Can you work these out from the model? Positions are in its coordinate system, mm. Face numbers are marked on the shaded views. A direction names the side the tool comes from. Coordinates: 2 decimals unless noted, no trailing zeros. Write each loop counter-clockwise with the first axis right and the second up, starting at its lowest first coordinate (ties: lowest second). Pieces come first, ordered by that corner, then holes. Notation, with made-up numbers: (70.5, -25.5) - (85.5, -25.5) arc R24 ccw to (85.5, 10.5) - close; hole circle Ø7 at (35, 7). An arc over 180 degrees is marked (long way). One line per question, with ' | ' between items. Start each with the question number.
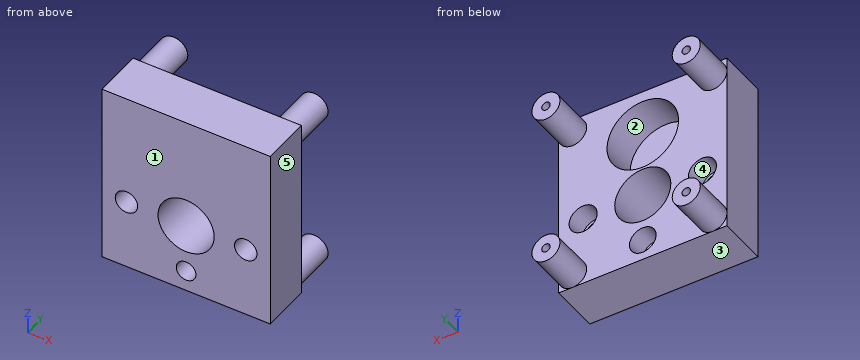
from build123d import *

# Parameters (mm, degrees)
SKETCH_1_W          = 12
SKETCH_1_H          = 13
SKETCH_1_R          = 2
SKETCH_1_R_2        = 0.8
SKETCH_1_R_3        = 0.7
EXTRUDE_1_DEPTH     = 3.5
CUT_EXTRUDE_START   = 3.5
SKETCH_1_3_R        = 1
SKETCH_1_3_R_2      = 0.95
CUT_EXTRUDE_2_DEPTH = 1.5
SKETCH_2_R          = 2.55
CUT_EXTRUDE_5_DEPTH = 2.6
SKETCH_3_R          = 1
EXTRUDE_2_DEPTH     = 3
CUT_EXTRUDE_START_2 = 3
SKETCH_3_3_R        = 0.3
CUT_EXTRUDE_6_DEPTH = 2


with BuildPart() as part:
    # 草图1 → 凸台-拉伸1 (new body)
    with BuildSketch(Plane(origin=(0, 0, 0), x_dir=(1, 0, 0), z_dir=(0, 1, 0))):
        with Locations((0, -1.5)):
            Rectangle(SKETCH_1_W, SKETCH_1_H)
        with Locations(Location((0, 0, 0), (0, 0, 270))):
            Circle(SKETCH_1_R, mode=Mode.SUBTRACT)
        with Locations(Location((-4.25, 0, 0), (0, 0, 270))):
            Circle(SKETCH_1_R_2, mode=Mode.SUBTRACT)
        with Locations(Location((4.25, 0, 0), (0, 0, 270))):
            Circle(SKETCH_1_R_2, mode=Mode.SUBTRACT)
        with Locations(Location((0, 3.5, 0), (0, 0, 270))):
            Circle(SKETCH_1_R_3, mode=Mode.SUBTRACT)
    extrude(amount=EXTRUDE_1_DEPTH)

    # 草图1<3> → 切除-拉伸2 (cut)
    with BuildSketch(Plane(origin=(0, 0, 0), x_dir=(1, 0, 0), z_dir=(0, 1, 0)).offset(CUT_EXTRUDE_START)):
        with Locations(Location((-4.25, 0, 0), (0, 0, 270))):
            Circle(SKETCH_1_3_R)
        with Locations(Location((4.25, 0, 0), (0, 0, 270))):
            Circle(SKETCH_1_3_R)
        with Locations(Location((0, 3.5, 0), (0, 0, 270))):
            Circle(SKETCH_1_3_R_2)
    extrude(amount=-CUT_EXTRUDE_2_DEPTH, mode=Mode.SUBTRACT)

    # 草图2 → 切除-拉伸5 (cut)
    with BuildSketch(Plane(origin=(0, 3.5, 0), x_dir=(1, 0, 0), z_dir=(0, 1, 0))):
        with Locations(Location((0, -4.7, 0), (0, 0, 270))):
            Circle(SKETCH_2_R)
    extrude(amount=-CUT_EXTRUDE_5_DEPTH, mode=Mode.SUBTRACT)

    # 草图3 → 凸台-拉伸2 (add)
    with BuildSketch(Plane(origin=(0, 3.5, 0), x_dir=(1, 0, 0), z_dir=(0, 1, 0))):
        with Locations(Location((-5, -7, 0), (0, 0, 270))):
            Circle(SKETCH_3_R)
        with Locations(Location((5, 4, 0), (0, 0, 90))):
            Circle(SKETCH_3_R)
        with Locations(Location((-5, 4, 0), (0, 0, 90))):
            Circle(SKETCH_3_R)
        with Locations(Location((5, -7, 0), (0, 0, 270))):
            Circle(SKETCH_3_R)
    extrude(amount=EXTRUDE_2_DEPTH)

    # 草图3<3> → 切除-拉伸6 (cut)
    with BuildSketch(Plane(origin=(0, 3.5, 0), x_dir=(1, 0, 0), z_dir=(0, 1, 0)).offset(CUT_EXTRUDE_START_2)):
        with Locations(Location((5, 4, 0), (0, 0, 270))):
            Circle(SKETCH_3_3_R)
        with Locations(Location((-5, -7, 0), (0, 0, 270))):
            Circle(SKETCH_3_3_R)
        with Locations(Location((-5, 4, 0), (0, 0, 270))):
            Circle(SKETCH_3_3_R)
        with Locations(Location((5, -7, 0), (0, 0, 270))):
            Circle(SKETCH_3_3_R)
    extrude(amount=-CUT_EXTRUDE_6_DEPTH, mode=Mode.SUBTRACT)


solid = part.part
(1) Which directions (+Z, -Z, +X, -X, +Y, -Y) give clear straight access to the entire face, cutting with the end or side of a thin tool? Please do the marked faces 1 and 2.
(2) If we section it at D-D on y = 3.25: List the corners of the cut face in (x, z) for me.
(3) If we section it at A-A on x = 0: List the corners of the cut face in (y, z) for me.
(4) If we mould it in two halves opening along X, with no side actions, what happens to the marked faces 3, 4 and 5? For each: +X half, -X half, draft (parallel to the pull), parting line (faces both ways), or undercut.
(5) If I drill on probe 1 along X at (y, z) = (0.8, 0); probe 2 along X at (y, z) = (5.9, -4); probe 3 along Z at (x, y) = (-4.25, 1.5), over which ranges is the centre line in solid material (lowest first)?
(6) If we section it at B-B on y = 5.75: List the corners of the cut face in (x, z) for me, plus the area to 3 significant figures.
(7) I'm going to push flat-ended pins straight in: pin 1 (0.6 mm diameter, centred on x = 0.5, z = -3.5, fed in from +Y); pin 2 (6 mm diameter, centred on x = 0, z = 4.7, fed in from +Y); pin 3 (0.5 mm diameter, centred on x = 5, z = -4, fed in from +Y). Where does each tip first touch, or does it pass through?
(8) If we section it at C-C on z = -3.5: List the corners of the cut face in (x, y) for me.
Values:
1) face 1: +Z, -Z, +X, -X, -Y | face 2: +Y
2) outline: (-6, -5) - (6, -5) - (6, 8) - (-6, 8) - close; hole circle Ø2 at (-4.25, 0); hole circle Ø5.1 at (0, 4.7); hole circle Ø4 at (0, 0); hole circle Ø1.9 at (0, -3.5); hole circle Ø2 at (4.25, 0)
3) outline: (0, -5) - (3.5, -5) - (3.5, -4.45) - (2, -4.45) - (2, -4.2) - (0, -4.2) - close; (0, -2.8) - (2, -2.8) - (2, -2.55) - (3.5, -2.55) - (3.5, -2) - (0, -2) - close; (0, 2) - (3.5, 2) - (3.5, 2.15) - (0.9, 2.15) - (0.9, 7.25) - (3.5, 7.25) - (3.5, 8) - (0, 8) - close
4) face 3: draft | face 4: undercut | face 5: +X half
5) probe 1: -6 to -5.05, -3.45 to -2, 2 to 3.45, 5.05 to 6 | probe 2: -6 to -5.3, -4.7 to -4, 4 to 4.7, 5.3 to 6 | probe 3: -5 to -0.8, 0.8 to 8
6) outline: circle Ø2 at (-5, -4); circle Ø2 at (-5, 7); circle Ø2 at (5, -4); circle Ø2 at (5, 7); hole circle Ø0.6 at (-5, -4); hole circle Ø0.6 at (-5, 7); hole circle Ø0.6 at (5, -4); hole circle Ø0.6 at (5, 7) | area: 11.4 mm2
7) pin 1: y = 2 | pin 2: y = 3.5 | pin 3: y = 4.5
8) outline: (-6, 0) - (-0.7, 0) - (-0.7, 2) - (-0.95, 2) - (-0.95, 3.5) - (-4.13, 3.5) - (-4.13, 6.5) - (-5.87, 6.5) - (-5.87, 3.5) - (-6, 3.5) - close; (0.7, 0) - (6, 0) - (6, 3.5) - (5.87, 3.5) - (5.87, 6.5) - (4.13, 6.5) - (4.13, 3.5) - (0.95, 3.5) - (0.95, 2) - (0.7, 2) - close
